```python
from build123d import *

# Parameters (mm, degrees)
F1_DEPTH = 150
F2_R     = 16.95362
F2_R_2   = 16.889789
F3_DEPTH = 100


with BuildPart() as f1:
    # F0 (on Front) → F1 (new body)
    with BuildSketch(Plane.XZ):
        Polygon((0, 90), (0, 0), (2, 0), (2, 88), (98, 88), (98, 0), (100, 0), (100, 90), align=None)
    extrude(amount=F1_DEPTH)

    # F2 (on face) → F3 (cut)
    with BuildSketch(Plane.YZ.offset(100)):
        with Locations((-126.991346, 52.532315)):
            Circle(F2_R)
        with Locations((-37.705854, 61.718065)):
            Circle(F2_R_2)
        Polygon((-78.490585, 28.893651), (-78.490585, 49.716024), (-98.293838, 56.150491), (-110.532922, 39.304838), (-98.293838, 22.459184), align=None)
    extrude(amount=-F3_DEPTH, mode=Mode.SUBTRACT)


solid = f1.part
```
Build history of the part. All positions in model axes, mm. A direction names the side the tool comes from. Give positions to 0.01 mm unless a question says otherwise; leave off trailing zeros. Loops run counter-clockwise (first coordinate to the right, second up) from the corner with the lowest first, then second, coordinate; pieces in that order, holes last.
1) Band-saw the part on D-D on y = -13. List the corners of the cut face in (x, z).
Values follow:
outline: (0, 0) - (2, 0) - (2, 88) - (98, 88) - (98, 0) - (100, 0) - (100, 90) - (0, 90) - close
2) Probe line 1 along X through (y, z) = (-104.5, 66); line 2 along Z through (x, y) = (79.5, -130). List the from-to ranges inside material, lowest first.
Values follow:
line 1: x = 0 to 2, 98 to 100
line 2: z = 88 to 90
3) Drop a flat-ended pin along its axis: P1, Ø8, axis at x = 47.5, y = -26.5, coming from the -Z side. Give the stop position or say it passes through.
Values follow:
P1: stops at z = 88
4) Two-plate mould, pull along Y, no slides. Class faces 1 (the face through (1.014, -88.254, 52.888)), 2 (the face through (99.01, -110.82, 57.62)), 3 (the face through (28, 0, 89)), 4 (the face through (51, -74, 90)): released by +Y, released by -Y, zero draft, split by the parting line, or undercut.
Values follow:
face 1: undercut
face 2: undercut
face 3: released by +Y
face 4: zero draft
5) Band-saw the part on B-B on y = -116.5. List the corners of the cut face in (x, z).
Values follow:
outline: (0, 0) - (2, 0) - (2, 39.21) - (0, 39.21) - close; (0, 65.85) - (2, 65.85) - (2, 88) - (98, 88) - (98, 65.85) - (100, 65.85) - (100, 90) - (0, 90) - close; (98, 0) - (100, 0) - (100, 39.21) - (98, 39.21) - close
6) 3-axis set-ups, long thin cutter, end or side, ignore diameter. For faces 5 (the face through (28, -150, 89)), 6 (the face through (2, -74, 43)), 7 (the face through (1.014, -104.328, 47.846)): which of +Z, -Z, +X, -X, +Y, -Y reach the whole face in a straight line?
Values follow:
face 5: +Z, -Z, +X, -X, -Y
face 6: -Z, +Y, -Y
face 7: +X, -X
7) Band-saw the part on C-C on z = 31. List the corners of the cut face in (x, y), then the cut area to 3 significant figures.
Values follow:
outline: (0, -150) - (2, -150) - (2, -104.5) - (0, -104.5) - close; (0, -78.49) - (2, -78.49) - (2, 0) - (0, 0) - close; (98, -150) - (100, -150) - (100, -104.5) - (98, -104.5) - close; (98, -78.49) - (100, -78.49) - (100, 0) - (98, 0) - close
area: 496 mm2
8) Band-saw the part on A-A on z = 6. List the corners of the cut face in (x, y).
Values follow:
outline: (0, -150) - (2, -150) - (2, 0) - (0, 0) - close; (98, -150) - (100, -150) - (100, 0) - (98, 0) - close
